Solid Edge part; units mm, degrees
sketch "Sketch1" plane through (0, 0, 0) normal (0, 0, 1) x (1, 0, 0)
  line L0 (-6.5, -8.5) -> (6.5, -8.5)
  line L1 (6.5, -8.5) -> (6.5, 8.5)
  line L2 (6.5, 8.5) -> (-6.5, 8.5)
  line L3 (-6.5, 8.5) -> (-6.5, -8.5)
extrude "Protrusion1" add sketch "Sketch1" along normal blind 25
sketch "Sketch2" plane through (0, 0, 25) normal (0, 0, 1) x (1, 0, 0)
  line L0 (0, 0) -> (6.5, -6.2249)
  line L1 (6.5, 6.2249) -> (6.5, -6.2249)
  line L2 (0, 0) -> (6.5, 6.2249)
extrude "ExtrudedCutout_1" cut sketch "Sketch2" against normal blind 29.2025
chamfer "Chamfer_1" distance 0.5 angle 45 14 edges at (3.25, 3.1125, 25) (3.25, -3.1125, 25) (6.5, 7.3625, 25) (0, 8.5, 25) (-6.5, 0, 25) (0, -8.5, 25) (6.5, -7.3625, 25) (0, -8.5, 0) (6.5, -7.3625, 0) (3.25, -3.1125, 0) (3.25, 3.1125, 0) (6.5, 7.3625, 0) (0, 8.5, 0) (-6.5, 0, 0)
Can you work these out from the model? Positions are in its coordinate system, mm. A direction names the side the tool comes from. Round coordinates to 2 decimals unless told otherwise and drop trailing zeros. Write each loop counter-clockwise with the first axis right and the second up, starting at its lowest first coordinate (ties: lowest second). Pieces come first, ordered by that corner, then holes. Notation, with made-up numbers: M 25,46 L 83,46 A6 cw 83,54 Z; hole C -6,9.5 d2. An arc over 180 degrees is marked long. Use a Markdown table: item, result.
Item 1: I want a section at B-B (z = 12.75). List the corners of the cut face in (x, y) for me, and give its area (3 significant figures).
Found:
| item | result |
|---|---|
| outline | M -6.5,-8.5 L 6.5,-8.5 L 6.5,-6.22 L 0,0 L 6.5,6.22 L 6.5,8.5 L -6.5,8.5 Z |
| area | 181 mm2 |
Item 2: I want a section at D-D (y = -1.25). List the corners of the cut face in (x, z) for me.
Found:
| item | result |
|---|---|
| outline | M -6.5,0.5 L -6,0 L 0.58,0 L 1.31,0.5 L 1.31,24.5 L 0.58,25 L -6,25 L -6.5,24.5 Z |
Item 3: If I drill on line 1 along Y through (x, z) = (1.25, 5.25); line 2 along Y through (x, z) = (1, 18.25); line 3 along X through (y, z) = (-5.75, 11), over which ranges is the centre line in solid material (lowest first)? Write a range as [from, to].
Found:
| item | result |
|---|---|
| line 1 | y = [-8.5, -1.2], [1.2, 8.5] |
| line 2 | y = [-8.5, -0.96], [0.96, 8.5] |
| line 3 | x = [-6.5, 6] |
Item 4: We'd pull the mould along Y, two halves only. Please class faces 5 (the face through (0, 8.5, 12)), 6 (the face through (3.204, 3.069, 12.668)), 7 (the face through (6.5, -7, 12)): released by +Y, released by -Y, zero draft, split by the parting line, or undercut.
Found:
| item | result |
|---|---|
| face 5 | released by +Y |
| face 6 | undercut |
| face 7 | zero draft |
Item 5: For pin 1 Ø3 at (y, z) = (4.5, 6.5) entering from +X; pin 2 Ø8 at (y, z) = (-5.5, 14.5) entering from +X, each with a flat end and sliding along its axis, tell me the tip position at first contact or that it passes through.
Found:
| item | result |
|---|---|
| pin 1 | stops at x = 6.27 |
| pin 2 | stops at x = 6.5 |
Item 6: I want a section at A-A (x = 4). List the corners of the cut face in (y, z) for me.
Found:
| item | result |
|---|---|
| outline | M -8.5,0.5 L -8,0 L -4.52,0 L -3.83,0.5 L -3.83,24.5 L -4.52,25 L -8,25 L -8.5,24.5 Z; M 3.83,0.5 L 4.52,0 L 8,0 L 8.5,0.5 L 8.5,24.5 L 8,25 L 4.52,25 L 3.83,24.5 Z |
Item 7: I want a section at C-C (y = -3). List the corners of the cut face in (x, z) for me, and give its area (3 significant figures).
Found:
| item | result |
|---|---|
| outline | M -6.5,0.5 L -6,0 L 2.41,0 L 3.13,0.5 L 3.13,24.5 L 2.41,25 L -6,25 L -6.5,24.5 Z |
| area | 240 mm2 |
Item 8: Which directions (+Z, -Z, +X, -X, +Y, -Y) give clear straight access to the entire face, cutting with the end or side of a thin tool? Please do faces 1 (the face through (3.204, -3.069, 12.668)), 2 (the face through (2.94, 3.16, 24.75)), 3 (the face through (2.94, 3.16, 0.25)), 4 (the face through (0, -8.5, 12)).
Found:
| item | result |
|---|---|
| face 1 | +Z, -Z, +X |
| face 2 | +Z, +X |
| face 3 | -Z, +X |
| face 4 | +Z, -Z, +X, -X, -Y |
